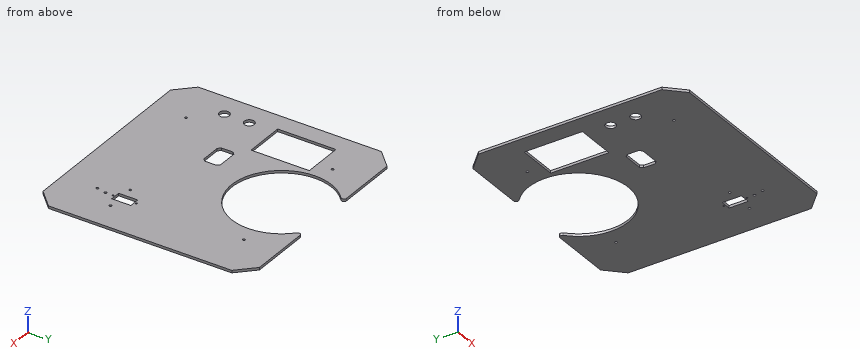
from build123d import *

# Parameters (mm, degrees)
SKETCH_1_W          = 270
SKETCH_1_H          = 260
EXTRUDE_1_DEPTH     = 3
CHAMFER_2_SIZE      = 20
SKETCH_4_R          = 60
CUT_EXTRUDE_1_DEPTH = 10
FILLET_1_R          = 3
SKETCH_5_R          = 1.5
SKETCH_5_R_2        = 1.05
SKETCH_5_W          = 12.5
SKETCH_5_H          = 23.002638066
CUT_EXTRUDE_2_DEPTH = 10
SKETCH_6_W          = 48
SKETCH_6_H          = 70
CUT_EXTRUDE_3_DEPTH = 0.1
SKETCH_10_W         = 48
SKETCH_10_H         = 70
CUT_EXTRUDE_4_DEPTH = 188.440657276
SKETCH_11_R         = 6
CUT_EXTRUDE_5_DEPTH = 188.440657276
SKETCH_13_R         = 1.5
CUT_EXTRUDE_6_DEPTH = 188.440657276
SKETCH_15_W         = 30
SKETCH_15_H         = 20
CUT_EXTRUDE_8_DEPTH = 188.440657276
CHAMFER_4_SIZE      = 3


with BuildPart() as part:
    # 草图1 → 凸台-拉伸1 (new body)
    with BuildSketch(Plane.XY):
        Rectangle(SKETCH_1_W, SKETCH_1_H)
    extrude(amount=EXTRUDE_1_DEPTH)

    # 倒角2
    chamfer_2_edges = [part.edges().sort_by_distance(p)[0] for p in [
        (135, -130, 1.5),
        (-135, -130, 1.5),
        (-135, 130, 1.5),
        (135, 130, 1.5),
    ]]
    chamfer(chamfer_2_edges, length=CHAMFER_2_SIZE)

    # 草图4 → 切除-拉伸1 (cut)
    with BuildSketch(Plane.XY.offset(3)):
        with Locations((0, 80)):
            Circle(SKETCH_4_R)
    extrude(amount=-CUT_EXTRUDE_1_DEPTH, mode=Mode.SUBTRACT)

    # 圆角1
    fillet_1_edges = [part.edges().sort_by_distance(p)[0] for p in [
        (33.166247904, 130, 1.5),
        (-33.166247904, 130, 1.5),
    ]]
    fillet(fillet_1_edges, radius=FILLET_1_R)

    # 草图5 → 切除-拉伸2 (cut)
    with BuildSketch(Plane(origin=(0, 0, 0), x_dir=(-1, 0, 0), z_dir=(0, 0, -1))):
        with Locations((-64.7, -58.75)):
            Circle(SKETCH_5_R)
        with Locations((-100.3, -58.75)):
            Circle(SKETCH_5_R)
        with Locations((-82.5, -76.55)):
            Circle(SKETCH_5_R)
        with Locations((-82.5, -39.65)):
            Circle(SKETCH_5_R_2)
        with Locations((-82.5, -67.35)):
            Circle(SKETCH_5_R_2)
        with Locations((-82.5, -53.445792921)):
            Rectangle(SKETCH_5_W, SKETCH_5_H)
    extrude(amount=-CUT_EXTRUDE_2_DEPTH, mode=Mode.SUBTRACT)

    # 草图6 → 切除-拉伸3 (cut)
    with BuildSketch(Plane(origin=(0, 0, 0), x_dir=(-1, 0, 0), z_dir=(0, 0, -1))):
        with Locations((89, 35)):
            Rectangle(SKETCH_6_W, SKETCH_6_H)
    extrude(amount=-CUT_EXTRUDE_3_DEPTH, mode=Mode.SUBTRACT)

    # 草图10 → 切除-拉伸4 (cut, through all)
    with BuildSketch(Plane(origin=(0, 0, 0), x_dir=(-1, 0, 0), z_dir=(0, 0, -1))):
        with Locations((89, 35)):
            Rectangle(SKETCH_10_W, SKETCH_10_H)
    extrude(amount=-CUT_EXTRUDE_4_DEPTH, mode=Mode.SUBTRACT)

    # 草图11 → 切除-拉伸5 (cut, through all)
    with BuildSketch(Plane.XY.offset(3)):
        with Locations((-107, -30)):
            Circle(SKETCH_11_R)
        with Locations((-107, -60)):
            Circle(SKETCH_11_R)
    extrude(amount=-CUT_EXTRUDE_5_DEPTH, mode=Mode.SUBTRACT)

    # 草图13 → 切除-拉伸6 (cut, through all)
    with BuildSketch(Plane(origin=(0, 0, 0), x_dir=(-1, 0, 0), z_dir=(0, 0, -1))):
        with Locations((80, 88)):
            Circle(SKETCH_13_R)
        with Locations((80, -88)):
            Circle(SKETCH_13_R)
        with Locations((-80, -88)):
            Circle(SKETCH_13_R)
        with Locations((-80, 88)):
            Circle(SKETCH_13_R)
    extrude(amount=-CUT_EXTRUDE_6_DEPTH, mode=Mode.SUBTRACT)

    # 草图15 → 切除-拉伸8 (cut, through all)
    with BuildSketch(Plane(origin=(0, 0, 0), x_dir=(-1, 0, 0), z_dir=(0, 0, -1))):
        with Locations((37, -20)):
            Rectangle(SKETCH_15_W, SKETCH_15_H)
    extrude(amount=-CUT_EXTRUDE_8_DEPTH, mode=Mode.SUBTRACT)

    # 倒角4
    chamfer_4_edges = [part.edges().sort_by_distance(p)[0] for p in [
        (-22, -30, 1.5),
        (-22, -10, 1.5),
        (-52, -10, 1.5),
        (-52, -30, 1.5),
    ]]
    chamfer(chamfer_4_edges, length=CHAMFER_4_SIZE)


solid = part.part
Build history of the part. All positions in model axes, mm. Round coordinates to 2 decimals unless told otherwise and drop trailing zeros. Write each loop counter-clockwise with the first axis right and the second up, starting at its lowest first coordinate (ties: lowest second). Pieces come first, ordered by that corner, then holes. Notation, with made-up numbers: M 49.5,71.25 L 104.5,71.25 A21 ccw 104.5,94.25 Z; hole C 73,89.25 d10. An arc over 180 degrees is marked long. Answer in a Markdown table with one row per item.
1. Saw through at D-D (x = -4). List the corners of the cut face in (y, z), and give its area (3 significant figures).
Geometry check:
| item | result |
|---|---|
| outline | M -130,0 L 20.13,0 L 20.13,3 L -130,3 Z |
| area | 450 mm2 |
2. Saw through at C-C (y = 106). List the corners of the cut face in (x, z), and give its area (3 significant figures).
Geometry check:
| item | result |
|---|---|
| outline | M -135,0 L -54.07,0 L -54.07,3 L -135,3 Z; M 54.07,0 L 135,0 L 135,3 L 54.07,3 Z |
| area | 486 mm2 |
3. Saw through at A-A (y = -17.5). List the corners of the cut face in (x, z), and give its area (3 significant figures).
Geometry check:
| item | result |
|---|---|
| outline | M -135,0 L -52,0 L -52,3 L -135,3 Z; M -22,0 L 135,0 L 135,3 L -22,3 Z |
| area | 720 mm2 |
4. Saw through at B-B (x = -107). List the corners of the cut face in (y, z), and give its area (3 significant figures).
Geometry check:
| item | result |
|---|---|
| outline | M -130,0 L -66,0 L -66,3 L -130,3 Z; M -54,0 L -36,0 L -36,3 L -54,3 Z; M -24,0 L 0,0 L 0,3 L -24,3 Z; M 70,0 L 130,0 L 130,3 L 70,3 Z |
| area | 498 mm2 |
5. Probe L1, parallel to Y at x = -80, z = 1.75; L2, parallel to Y at x = 82.5, z = 0.85; L3, parallel to Y at x = -107, z = 0.95. List the from-to ranges inside material, lowest first. Write a range as [from, to].
Geometry check:
| item | result |
|---|---|
| L1 | [-130, -89.5], [-86.5, 0], [70, 86.5], [89.5, 130] |
| L2 | [-130, -78.05], [-75.05, -68.4], [-66.3, -64.95], [-41.94, -40.7], [-38.6, 130] |
| L3 | [-130, -66], [-54, -36], [-24, 0], [70, 130] |
